Verification items for the finished model (mm, model axes). A direction names the side the tool comes from. Round coordinates to 2 decimals unless told otherwise and drop trailing zeros. Order: outer loops, then holes, each group sorted by start corner. A loop starts at its lowest first (then second) coordinate and runs counter-clockwise, first axis right, second up. Notation, with made-up numbers: (29.25, 28) -> (63.25, 28) arc R21 cw to (63.25, 35) -> close; hole circle Ø10 at (21, -18). An arc over 180 degrees is marked (long way). Return JSON: item names as keys, results as strings. Group by question number.
Item 1: Scan lines: probe 1 along X at (y, z) = (4, 25); probe 2 along Y at (x, z) = (-5.5, -23); probe 3 along X at (y, z) = (6.95, -6.65). Record each from-to range of solid material in increasing order. Write a range as from..to.
Item 2: Depth check by flat-ended pin: pin 1 Ø1.3 at (y, z) = (8.5, 5.5) entering from -X; pin 2 Ø19 at (x, z) = (-4.5, 0) entering from +Y; pin 3 Ø3 at (x, y) = (9, 9.5) entering from +Z. Enter the tip coordinate at first touch or a pass-through.
Item 3: Sectioned sample at B-B on z = 25. Record the cut outline in (x, y).
Item 4: Draft check along Z on faces 4 (the flat face through (50, 2, 0)), 5 (the cylindrical face through (-42.373, 2.465, 21.905)), 6 (the cylindrical face through (-48.797, 2.465, -36.359)). Enter one of: pulls with the +Z half, pulls with the -Z half, needs draft (parallel to the pull), parting line crosses it, or undercut.
Item 5: Sectioned sample at D-D on y = 14.5. Record the cut outline in (x, z), plus the area to 3 significant figures.
Item 6: Access from +Z, -Z, +X, -X, +Y, -Y to the whole of each face (thin tool, end or side, straight path). Record for faces 1 (the flat face through (0, 5.4, 4)), 2 (the flat face through (4, 7.8, 1)), 3 (the cylindrical face through (-48.859, 2.465, 36.297)).
Item 7: Sectioned sample at C-C on x = 0. Give the number of separate pieces and of enclosed holes in the cut face, plus the area to 3 significant figures.
Item 8: Sectioned sample at A-A on x = 40. Record the cut outline in (y, z).
```python
from build123d import *

# Parameters (mm, degrees)
ESQUISSE1_R             = 3.9
BOSS_EXTRU_1_DEPTH      = 5
ESQUISSE2_R             = 23
ESQUISSE2_R_2           = 19
BOSS_EXTRU_2_DEPTH      = 12
ESQUISSE5_R             = 19
BOSS_EXTRU_3_DEPTH      = 4
ENL_V_MAT_EXTRU_4_DEPTH = 1.2
ESQUISSE9_R             = 3.55
ENL_V_MAT_EXTRU_5_DEPTH = 64.173491276
ESQUISSE6_R             = 19
ENL_V_MAT_EXTRU_3_DEPTH = 5.4
ESQUISSE10_R            = 1.1
ESQUISSE10_R_2          = 0.5
ENL_V_MAT_EXTRU_6_DEPTH = 64.173491276


with BuildPart() as part:
    # Esquisse1 → Boss.-Extru.1 (new body)
    with BuildSketch(Plane(origin=(0, 0, 0), x_dir=(1, 0, 0), z_dir=(0, 1, 0))):
        with BuildLine():
            Line((46, 37.5), (-46, 37.5))
            ThreePointArc((-46, 37.5), (-48.828427125, 36.328427125), (-50, 33.5))
            Line((-50, 33.5), (-50, -33.5))
            ThreePointArc((-50, -33.5), (-48.828427125, -36.328427125), (-46, -37.5))
            Line((-46, -37.5), (46, -37.5))
            ThreePointArc((46, -37.5), (48.828427125, -36.328427125), (50, -33.5))
            Line((50, -33.5), (50, 33.5))
            ThreePointArc((50, 33.5), (48.828427125, 36.328427125), (46, 37.5))
        make_face()
        with Locations(Location((-40, -25, 0), (0, 0, 270))):
            Circle(ESQUISSE1_R, mode=Mode.SUBTRACT)
        with Locations(Location((40, -25, 0), (0, 0, 270))):
            Circle(ESQUISSE1_R, mode=Mode.SUBTRACT)
        with Locations(Location((-40, 25, 0), (0, 0, 270))):
            Circle(ESQUISSE1_R, mode=Mode.SUBTRACT)
        with Locations(Location((40, 25, 0), (0, 0, 270))):
            Circle(ESQUISSE1_R, mode=Mode.SUBTRACT)
    extrude(amount=BOSS_EXTRU_1_DEPTH)

    # Esquisse2 → Boss.-Extru.2 (add)
    with BuildSketch(Plane(origin=(0, 5, 0), x_dir=(1, 0, 0), z_dir=(0, 1, 0))):
        with Locations(Location((0, 0, 0), (0, 0, 270))):
            Circle(ESQUISSE2_R)
        with Locations(Location((0, 0, 0), (0, 0, 270))):
            Circle(ESQUISSE2_R_2, mode=Mode.SUBTRACT)
    extrude(amount=BOSS_EXTRU_2_DEPTH)

    # Esquisse5 → Boss.-Extru.3 (add)
    with BuildSketch(Plane(origin=(0, 5, 0), x_dir=(1, 0, 0), z_dir=(0, 1, 0))):
        with Locations(Location((0, 0, 0), (0, 0, 270))):
            Circle(ESQUISSE5_R)
    extrude(amount=BOSS_EXTRU_3_DEPTH)

    # Esquisse8 → Enlèv. mat.-Extru.4 (cut)
    with BuildSketch(Plane(origin=(0, 9, 0), x_dir=(1, 0, 0), z_dir=(0, 1, 0))):
        with BuildLine():
            Line((2.25, -6.3), (2.25, -3.145492982))
            Line((2.25, -3.145492982), (16.35, -1.8))
            ThreePointArc((16.35, -1.8), (18.15, 0), (16.35, 1.8))
            Line((16.35, 1.8), (2.25, 3.145492982))
            Line((2.25, 3.145492982), (2.25, 6.3))
            ThreePointArc((2.25, 6.3), (0, 8.55), (-2.25, 6.3))
            Line((-2.25, 6.3), (-2.25, 3.264730494))
            Line((-2.25, 3.264730494), (-13.769370638, 2.199914721))
            ThreePointArc((-13.769370638, 2.199914721), (-15.95, 0), (-13.769370638, -2.199914721))
            Line((-13.769370638, -2.199914721), (-2.25, -3.264730494))
            Line((-2.25, -3.264730494), (-2.25, -6.3))
            ThreePointArc((-2.25, -6.3), (0, -8.55), (2.25, -6.3))
        make_face()
    extrude(amount=-ENL_V_MAT_EXTRU_4_DEPTH, mode=Mode.SUBTRACT)

    # Esquisse9 → Enlèv. mat.-Extru.5 (cut, through all)
    with BuildSketch(Plane(origin=(0, 7.8, 0), x_dir=(1, 0, 0), z_dir=(0, 1, 0))):
        with Locations(Location((0, 0, 0), (0, 0, 270))):
            Circle(ESQUISSE9_R)
    extrude(amount=-ENL_V_MAT_EXTRU_5_DEPTH, mode=Mode.SUBTRACT)

    # Esquisse6 → Enlèv. mat.-Extru.3 (cut)
    with BuildSketch(Plane.XZ):
        with Locations(Location((0, 0, 0), (0, 0, 90))):
            Circle(ESQUISSE6_R)
    extrude(amount=-ENL_V_MAT_EXTRU_3_DEPTH, mode=Mode.SUBTRACT)

    # Esquisse10 → Enlèv. mat.-Extru.6 (cut, through all)
    # profile 1 of 10: a face of its own
    with BuildSketch(Plane(origin=(0, 7.8, 0), x_dir=(1, 0, 0), z_dir=(0, 1, 0))):
        with Locations(Location((0, 6.65, 0), (0, 0, 270))):
            Circle(ESQUISSE10_R)
        with Locations((0, 6.65)):
            Circle(ESQUISSE10_R_2, mode=Mode.SUBTRACT)
    # profile 2 of 10: a face of its own
    with BuildSketch(Plane(origin=(0, 7.8, 0), x_dir=(1, 0, 0), z_dir=(0, 1, 0))):
        with Locations((0, 6.65)):
            Circle(ESQUISSE10_R_2)
    # profile 3 of 10: a face of its own
    with BuildSketch(Plane(origin=(0, 7.8, 0), x_dir=(1, 0, 0), z_dir=(0, 1, 0))):
        with Locations(Location((0, -6.65, 0), (0, 0, 270))):
            Circle(ESQUISSE10_R)
        with Locations((0, -6.65)):
            Circle(ESQUISSE10_R_2, mode=Mode.SUBTRACT)
    # profile 4 of 10: a face of its own
    with BuildSketch(Plane(origin=(0, 7.8, 0), x_dir=(1, 0, 0), z_dir=(0, 1, 0))):
        with Locations((0, -6.65)):
            Circle(ESQUISSE10_R_2)
    # profile 5 of 10: a face of its own
    with BuildSketch(Plane(origin=(0, 7.8, 0), x_dir=(1, 0, 0), z_dir=(0, 1, 0))):
        with Locations(Location((-8.19, 0, 0), (0, 0, 270))):
            Circle(ESQUISSE10_R)
        with Locations((-8.19, 0)):
            Circle(ESQUISSE10_R_2, mode=Mode.SUBTRACT)
    # profile 6 of 10: a face of its own
    with BuildSketch(Plane(origin=(0, 7.8, 0), x_dir=(1, 0, 0), z_dir=(0, 1, 0))):
        with Locations((-8.19, 0)):
            Circle(ESQUISSE10_R_2)
    # profile 7 of 10: a face of its own
    with BuildSketch(Plane(origin=(0, 7.8, 0), x_dir=(1, 0, 0), z_dir=(0, 1, 0))):
        with Locations(Location((6.8, 0, 0), (0, 0, 270))):
            Circle(ESQUISSE10_R)
        with Locations((6.8, 0)):
            Circle(ESQUISSE10_R_2, mode=Mode.SUBTRACT)
    # profile 8 of 10: a face of its own
    with BuildSketch(Plane(origin=(0, 7.8, 0), x_dir=(1, 0, 0), z_dir=(0, 1, 0))):
        with Locations((6.8, 0)):
            Circle(ESQUISSE10_R_2)
    # profile 9 of 10: a face of its own
    with BuildSketch(Plane(origin=(0, 7.8, 0), x_dir=(1, 0, 0), z_dir=(0, 1, 0))):
        with Locations(Location((12.65, 0, 0), (0, 0, 270))):
            Circle(ESQUISSE10_R)
        with Locations((12.65, 0)):
            Circle(ESQUISSE10_R_2, mode=Mode.SUBTRACT)
    # profile 10 of 10: a face of its own
    with BuildSketch(Plane(origin=(0, 7.8, 0), x_dir=(1, 0, 0), z_dir=(0, 1, 0))):
        with Locations((12.65, 0)):
            Circle(ESQUISSE10_R_2)
    extrude(amount=-ENL_V_MAT_EXTRU_6_DEPTH, mode=Mode.SUBTRACT)


solid = part.part
```
Recorded:
{
 "1": {"probe 1": "-50..-43.9, -36.1..36.1, 43.9..50", "probe 2": "0..5", "probe 3": "-22.02..-1.1, 1.1..22.02"},
 "2": {"pin 1": "x = -22.48", "pin 2": "y = 9", "pin 3": "z = 21.74"},
 "3": {"outline": "(-50, 0) -> (-43.9, 0) -> (-43.9, 5) -> (-50, 5) -> close; (-36.1, 0) -> (36.1, 0) -> (36.1, 5) -> (-36.1, 5) -> close; (43.9, 0) -> (50, 0) -> (50, 5) -> (43.9, 5) -> close"},
 "4": {"face 4": "needs draft", "face 5": "undercut", "face 6": "pulls with the -Z half"},
 "5": {"outline": "circle Ø46 at (0, 0); hole circle Ø38 at (0, 0)", "area": "528 mm²"},
 "6": {"face 1": "-Y", "face 2": "+Y", "face 3": "+Z, -X, +Y, -Y"},
 "7": {"separate pieces": "4", "enclosed holes": "0", "area": "370 mm²"},
 "8": {"outline": "(0, -37.5) -> (5, -37.5) -> (5, -28.9) -> (0, -28.9) -> close; (0, -21.1) -> (5, -21.1) -> (5, 21.1) -> (0, 21.1) -> close; (0, 28.9) -> (5, 28.9) -> (5, 37.5) -> (0, 37.5) -> close"}
}
